Check sheet for the modelled part. Datum: model origin and axes. Units: mm. A direction names the side the tool comes from. Coordinates: 2 decimals unless noted, no trailing zeros. Order: outer loops, then holes, each group sorted by start corner. A loop starts at its lowest first (then second) coordinate and runs counter-clockwise, first axis right, second up. Notation, with made-up numbers: (41, -35.5) -> (87, -35.5) arc R16 ccw to (87, -14.5) -> close; hole circle Ø3 at (45.25, 12.5). An arc over 180 degrees is marked (long way). Put each result on its own line as item: value. Start each with the question number.
Autodesk Inventor part; units mm, degrees
ref_plane "Work Plane2" through (228.6, 0, 6.35) normal (1, 0, 0) x (0, 0, -1)
ref_plane "YZ Plane" through (0, 0, 0) normal (1, 0, 0) x (0, 1, 0)
ref_plane "XZ Plane" through (0, 0, 0) normal (0, 1, 0) x (-1, 0, 0)
sketch "Sketch1" plane through (0, 0, 0) normal (0, 0, 1) x (1, 0, 0)
  line L0 (0, 0) -> (228.6, 0)
  line L1 (228.6, 0) -> (228.6, 469.9)
  line L2 (228.6, 469.9) -> (0, 469.9)
  line L3 (0, 469.9) -> (0, 0)
  dimension "d0" = 469.9
  dimension "d1" = 228.6
extrude "Extrusion1" add sketch "Sketch1" along normal blind 6.35
sketch "Sketch2" plane through (0, 0, 6.35) normal (0, 0, 1) x (1, 0, 0)
  line L0 (228.6, 469.9) -> (0, 469.9)
  line L1 (38.1, 469.9) -> (0, 431.8)
  line L2 (0, 469.9) -> (0, 0)
  line L3 (0, 88.9) -> (88.9, 0)
  line L4 (0, 0) -> (228.6, 0)
  line L5 (0, 88.9) -> (0, 0)
  line L6 (0, 0) -> (88.9, 0)
  line L7 (38.1, 469.9) -> (0, 469.9)
  line L8 (0, 431.8) -> (0, 469.9)
  circle A0 centre (12.7, 457.2) radius 2.54
  circle A1 centre (12.7, 431.8) radius 2.54
  circle A2 centre (12.7, 406.4) radius 2.54
  circle A3 centre (12.7, 381) radius 2.54
  circle A4 centre (12.7, 355.6) radius 2.54
  circle A5 centre (12.7, 330.2) radius 2.54
  circle A6 centre (12.7, 304.8) radius 2.54
  circle A7 centre (12.7, 279.4) radius 2.54
  circle A8 centre (12.7, 254) radius 2.54
  circle A9 centre (12.7, 228.6) radius 2.54
  circle A10 centre (12.7, 203.2) radius 2.54
  circle A11 centre (12.7, 177.8) radius 2.54
  circle A12 centre (12.7, 152.4) radius 2.54
  circle A13 centre (12.7, 127) radius 2.54
  circle A14 centre (12.7, 101.6) radius 2.54
  circle A15 centre (12.7, 76.2) radius 2.54
  circle A16 centre (12.7, 50.8) radius 2.54
  circle A17 centre (12.7, 25.4) radius 2.54
  line L9 (25.4, 444.5) -> (76.2, 444.5)
  line L10 (76.2, 444.5) -> (76.2, 368.3)
  line L11 (76.2, 368.3) -> (25.4, 368.3)
  line L12 (25.4, 368.3) -> (25.4, 444.5)
  line L13 (25.4, 355.6) -> (71.12, 355.6)
  line L14 (71.12, 355.6) -> (71.12, 254)
  line L15 (71.12, 254) -> (25.4, 254)
  line L16 (25.4, 254) -> (25.4, 355.6)
  line L17 (95.25, 444.5) -> (95.25, 368.3)
  line L18 (95.25, 368.3) -> (171.45, 368.3)
  line L19 (95.25, 444.5) -> (171.45, 368.3)
  line L20 (211.9249, 469.9) -> (211.9249, 50.8)
  line L21 (228.6, 0) -> (228.6, 469.9)
  line L22 (101.6, 469.9) -> (228.6, 342.9)
  line L23 (101.6, 469.9) -> (228.6, 469.9)
  line L24 (228.6, 469.9) -> (228.6, 342.9)
  line L25 (211.9249, 50.8) -> (228.6, 50.8)
  line L26 (228.6, 50.8) -> (228.6, 342.9)
  circle A18 centre (186.5249, 325.12) radius 17.78
  circle A19 centre (186.5249, 274.32) radius 17.78
  circle A20 centre (186.5249, 223.52) radius 17.78
  circle A21 centre (186.5249, 172.72) radius 17.78
  line L27 (211.9249, 359.5751) -> (228.6, 342.9)
  line L28 (211.9249, 359.5751) -> (211.9249, 50.8)
  line L29 (211.9249, 50.8) -> (228.6, 50.8)
  line L30 (228.6, 50.8) -> (228.6, 342.9)
  dimension "d4" = 38.1
  dimension "d5" = 38.1
  dimension "d6" = 88.9
  dimension "d7" = 0
  dimension "d8" = 88.9
  dimension "d9" = 5.08
  dimension "d10" = 12.7
  dimension "d11" = 12.7
  dimension "d14" = 25.4
  dimension "d20" = 50.8
  dimension "d21" = 76.2
  dimension "d22" = 25.4
  dimension "d23" = 25.4
  dimension "d24" = 45.72
  dimension "d25" = 101.6
  dimension "d27" = 25.4
  dimension "d28" = 19.05
  dimension "d29" = 76.2
  dimension "d30" = 76.2
  dimension "d31" = 0
  dimension "d32" = 12.7
  dimension "d33" = 16.6751
  dimension "d34" = 0
  dimension "d35" = 50.8
  dimension "d37" = 127
  dimension "d38" = 35.56
  dimension "d39" = 17.78
  dimension "d42" = 50.8
  dimension "d47" = 25.4
extrude "Extrusion2" cut sketch "Sketch2" against normal blind 25.4 contours L21 L22 L20 L0 | L20 L22 L0 | L21 L25 L20 L22 | L1 L2 L0 | L4 L2 L3 A15 | A15 L3 | A0 | A1 | A2 | A3 | A4 | A5 | A6 | A7 | A8 | A9 | A10 | A11 | A12 | A13 | A14 | A16 | A17 | L9 L10 L11 L12 | L13 L14 L15 L16 | L19 L18 L17 | A18 | A19 | A20 | A21 picked at (11.9754, 76.638)
ref_plane "Work Plane2" through (228.6, 0, 6.35) normal (1, 0, 0) x (0, 0, -1)
mirror "Mirror1" about plane through (228.6, 0, 6.35) normal (1, 0, 0) of "Extrusion1", "Extrusion2"
sketch "Sketch3" plane through (0, 0, 6.35) normal (0, 0, 1) x (1, 0, 0)
  circle A0 centre (12.7, 76.2) radius 2.54
  circle A1 centre (12.7, 101.6) radius 2.54
  line L0 (12.7, 76.2) -> (25.4, 76.2)
  line L1 (25.4, 76.2) -> (25.4, 63.5)
  line L2 (88.9, 0) -> (0, 88.9)
  line L3 (25.4, 63.5) -> (12.7, 76.2)
  circle A2 centre (444.5, 76.2) radius 2.54
  circle A3 centre (444.5, 101.6) radius 2.54
  line L4 (444.5, 76.2) -> (431.8, 76.2)
  line L5 (431.8, 76.2) -> (431.8, 63.5)
  line L6 (431.8, 63.5) -> (444.5, 76.2)
  line L7 (457.2, 88.9) -> (368.3, 0)
  point P0 (0, 0)
  dimension "d52" = 5.08
  dimension "d53" = 25.4
  dimension "d54" = 0
  dimension "d55" = 12.7
  dimension "d56" = 5.08
  dimension "d57" = 25.4
  dimension "d58" = 0
  dimension "d59" = 12.7
extrude "Extrusion3" cut sketch "Sketch3" against normal blind 25.4 contours L0 L1 L2 A0 | A0 L2 L0 | L6 L5 L4 A2 | A2 L4 L6 picked at (14.3126, 75.7108)
equation "\"d27\" = d23"
properties part number "Kermit Board" material "Glass"
1) Sectioned sample at A-A (x = 143.5). Record the boundary of the cut face in (y, z), plus the area to 3 significant figures.
2) Sectioned sample at B-B (z = 2.25). State how many separate pieces and enclosed holes the cut face has, plus the area to 3 significant figures.
3) Scan lines: line 1 along X through (y, z) = (298, 4.75); line 2 along X through (y, z) = (64.5, 3); line 3 along Y through (x, z) = (271, 3). Record each from-to range of solid material in increasing order. Write a range as [from, to].
4) Mould release check, pull along X, two halves, no side actions. Record for faces 4 (the cylindrical face through (288.438, 324.338, 3.219)), 5 (the flat face through (438, 451, 3)), 6 (the flat face through (175, 238, 6.35)): +X half, -X half, draft (parallel to the pull), parting line (faces both ways), or undercut.
5) Sectioned sample at C-C (x = 303.5). Record the boundary of the cut face in (y, z), plus the area to 3 significant figures.
6) Access from +Z, -Z, +X, -X, +Y, -Y to the whole of each face (thin tool, end or side, straight path). Record for faces 1 (the flat face through (175, 238, 0)), 2 (the flat face through (132.82, 406.93, 3.22)), 3 (the flat face through (156, 415.5, 3.2)).
7) Gauge pin test, flat ends, axial feed: pin 1 (1.5 mm diameter, centred on x = 110.5, z = 4.5, fed in from +Y); pin 2 (3 mm diameter, centred on x = 53, z = 2, fed in from -Y); pin 3 (1 mm diameter, centred on x = 350.5, z = 2, fed in from +Y). Record the tip position at first contact, or that the pin passes through.
Entries:
1. outline: (0, 0) -> (368.3, 0) -> (368.3, 6.35) -> (0, 6.35) -> close; (396.25, 0) -> (428, 0) -> (428, 6.35) -> (396.25, 6.35) -> close
1. area: 2,540 mm2
2. separate pieces: 1
2. enclosed holes: 42
2. area: 148,000 mm2
3. line 1: x = [0, 25.4], [71.12, 211.92], [245.28, 386.08], [431.8, 457.2]
3. line 2: x = [25.4, 211.92], [245.28, 431.8]
3. line 3: y = [0, 154.94], [190.5, 205.74], [241.3, 256.54], [292.1, 307.34], [342.9, 385.3]
4. face 4: undercut
4. face 5: +X half
4. face 6: draft
5. outline: (0, 0) -> (368.3, 0) -> (368.3, 6.35) -> (0, 6.35) -> close; (386.05, 0) -> (417.8, 0) -> (417.8, 6.35) -> (386.05, 6.35) -> close
5. area: 2,540 mm2
6. face 1: -Z, +X, -X, +Y, -Y
6. face 2: +Z, -Z
6. face 3: +Z, -Z, +Y
7. pin 1: stops at y = 461.75
7. pin 2: stops at y = 34.4
7. pin 3: stops at y = 465.3
